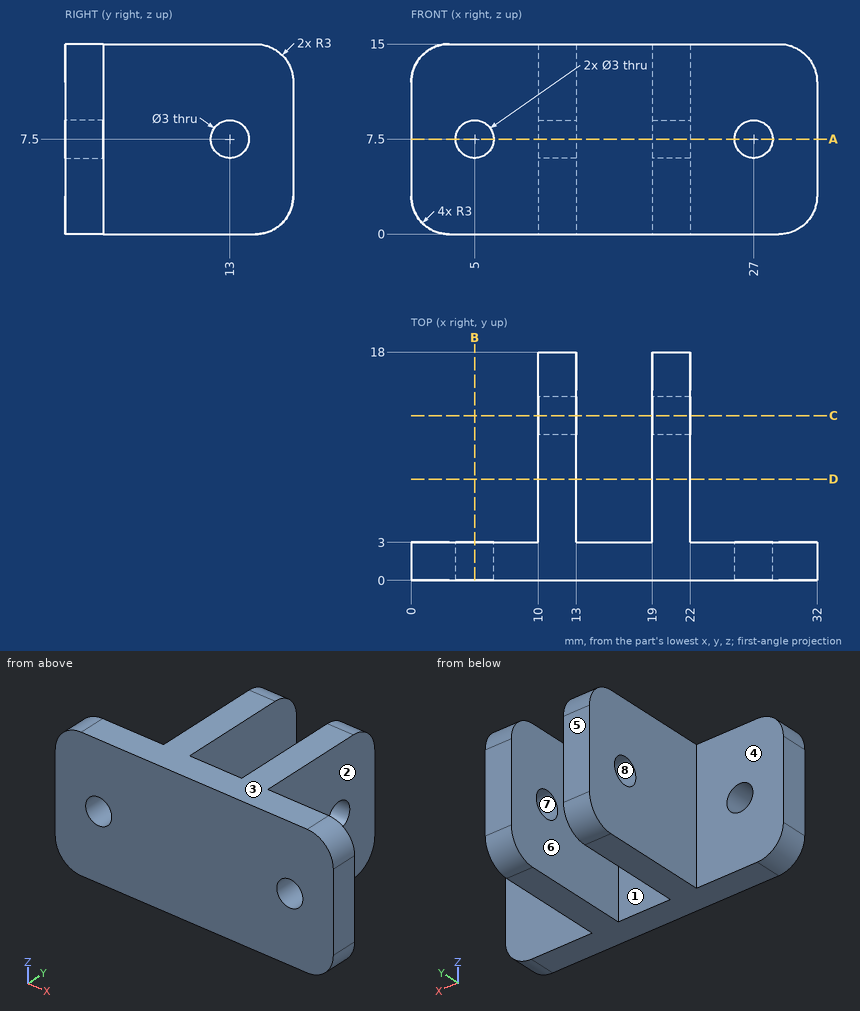
Source: three-view drawing plus pictorial views. Frame: mm from the lowest corner of the part. A direction names the side the tool comes from. Coordinates: 2 decimals unless noted, no trailing zeros. Loops run counter-clockwise (first coordinate to the right, second up) from the corner with the lowest first, then second, coordinate; pieces in that order, holes last. Notation, with made-up numbers: (32, 61) - (44, 61) arc R35 ccw to (44, 95) - close; hole circle Ø10 at (59, -39.5). An arc over 180 degrees is marked (long way). Answer in a Markdown table with one row per item. Add a question column.
Item 1: Contact query for flat-ended pins moving along their axis: P1, Ø3.5, axis at y = 13, z = 7.5, coming from the +X side; P2, Ø1.8, axis at x = 27, z = 7.5, coming from the +Y side (3 decimals); P3, Ø5, axis at y = 7.5, z = 3.5, coming from the -X side; P4, Ø3, axis at x = 5, z = 6.5, coming from the +Y side. Output: stop coordinate, or through.
Item 2: Section query D-D on y = 8. Return the cut outline in (x, z), then the cut area to 3 significant figures.
Item 3: Mould query, pull axis Y, two halves, no side actions, for the marked faces 5, 6, 7 and 8. Classes: released by +Y, released by -Y, zero draft, split by the parting line, or undercut.
Item 4: Section query B-B on x = 5. Return the cut outline in (y, z).
Item 5: Section query C-C on y = 13. Return the cut outline in (x, z), then the cut area to 3 significant figures.
Item 6: Access query for the marked faces 1, 2, 3 and 4. Directions: +Z, -Z, +X, -X, +Y, -Y. A direction counts if a zero-diameter tool reaches every point of the face in a straight line with its end or side. Return the directions, or none.
Item 7: Section query A-A on z = 7.5. Return the cut outline in (x, y).
Item 8: Line query: line 1 along X through (y, z) = (1.45, 7.5); line 2 along X through (y, z) = (16, 4.5); line 3 along Y through (x, z) = (20.95, 7.5). Output: solid intervals per line, ascending. Write a range as [from, to].
Recorded:
| question | item | result |
|---|---|---|
| 1 | P1 | x = 22 |
| 1 | P2 | through |
| 1 | P3 | x = 10 |
| 1 | P4 | y = 3 |
| 2 | outline | (10, 0) - (13, 0) - (13, 15) - (10, 15) - close; (19, 0) - (22, 0) - (22, 15) - (19, 15) - close |
| 2 | area | 90.0 mm^2 |
| 3 | face 5 | released by +Y |
| 3 | face 6 | zero draft |
| 3 | face 7 | undercut |
| 3 | face 8 | undercut |
| 4 | outline | (0, 0) - (3, 0) - (3, 6) - (0, 6) - close; (0, 9) - (3, 9) - (3, 15) - (0, 15) - close |
| 5 | outline | (10, 0) - (13, 0) - (13, 6) - (10, 6) - close; (10, 9) - (13, 9) - (13, 15) - (10, 15) - close; (19, 0) - (22, 0) - (22, 6) - (19, 6) - close; (19, 9) - (22, 9) - (22, 15) - (19, 15) - close |
| 5 | area | 72.0 mm^2 |
| 6 | face 1 | +Z, -Z, +Y |
| 6 | face 2 | +Z, -Z, +X, +Y |
| 6 | face 3 | +Z, +X, -X, +Y, -Y |
| 6 | face 4 | +Z, -Z, -X, +Y |
| 7 | outline | (0, 0) - (3.5, 0) - (3.5, 3) - (0, 3) - close; (6.5, 0) - (25.5, 0) - (25.5, 3) - (22, 3) - (22, 11.5) - (19, 11.5) - (19, 3) - (13, 3) - (13, 11.5) - (10, 11.5) - (10, 3) - (6.5, 3) - close; (10, 14.5) - (13, 14.5) - (13, 18) - (10, 18) - close; (19, 14.5) - (22, 14.5) - (22, 18) - (19, 18) - close; (28.5, 0) - (32, 0) - (32, 3) - (28.5, 3) - close |
| 8 | line 1 | [0, 3.5], [6.5, 25.5], [28.5, 32] |
| 8 | line 2 | [10, 13], [19, 22] |
| 8 | line 3 | [0, 11.5], [14.5, 18] |
